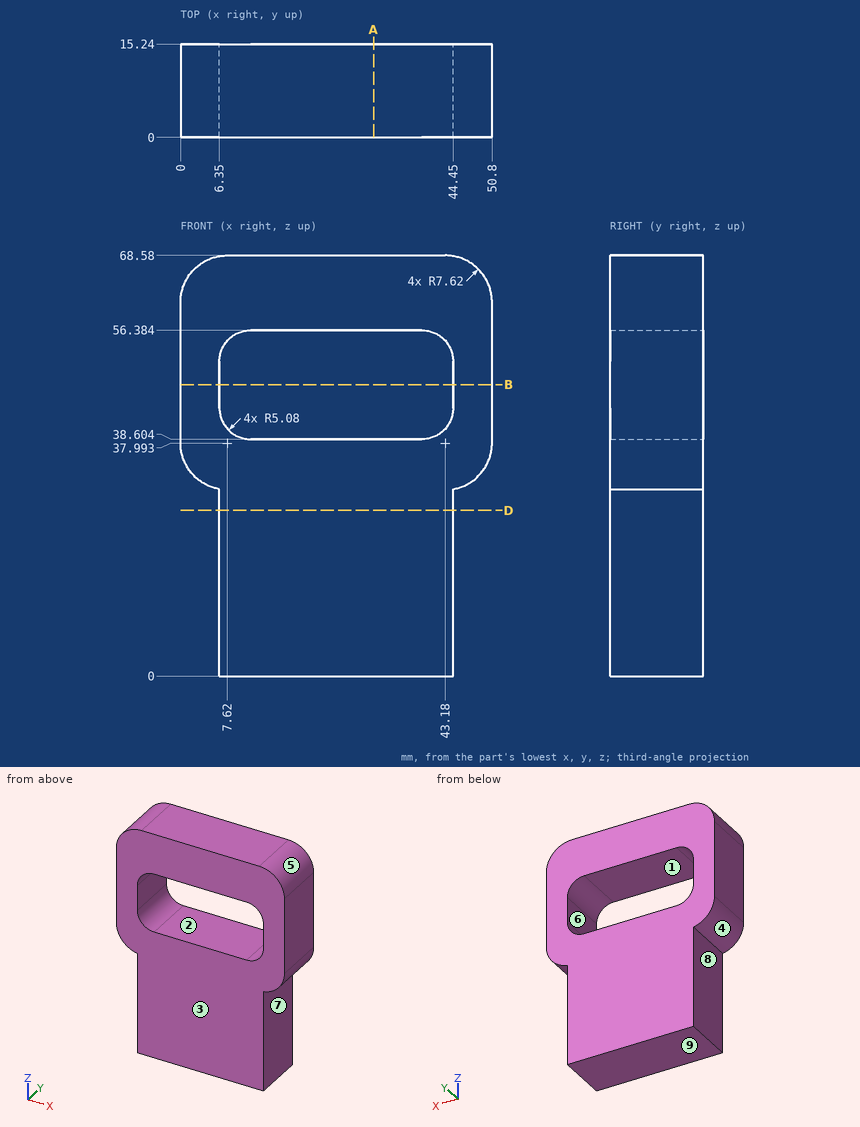
For this review, use the dimensioned drawing (mm, ordinates from the lowest corner) and the shaded views. A direction names the side the tool comes from. Give positions to 0.01 mm unless a question says otherwise; leave off trailing zeros. Loops run counter-clockwise (first coordinate to the right, second up) from the corner with the lowest first, then second, coordinate; pieces in that order, holes last. Notation, with made-up numbers: (64.25, -29) -> (82.25, -29) arc R12 cw to (82.25, -20) -> close; hole circle Ø4 at (78, 13). An arc over 180 degrees is marked (long way). Use CSV: the item, a comma, the result in double quotes.
1. Consider section D-D, the plane z = 27. Write out the cut boundary in (x, y).
Result:
outline,"(6.35, 0) -> (44.45, 0) -> (44.45, 15.24) -> (6.35, 15.24) -> close"
2. For P1, Ø5, axis at y = 5.5, z = 35, coming from the -X side; P2, Ø5, axis at x = 7.5, y = 5, coming from the -Z side; P3, Ø7.5, axis at y = 4, z = 18, coming from the +X side; P4, Ø1.5, axis at y = 11, z = 26, coming from the -X side, all flat-tipped, find the tip position at first contact; note any pin that passes through.
Result:
P1,"stops at x = 0.02"
P2,"stops at z = 0"
P3,"stops at x = 44.45"
P4,"stops at x = 6.35"
3. To check wall thickness, follow probe 1 along X at (y, z) = (14, 45); probe 2 along Z at (x, y) = (32.5, 2.25) (1 decimal); probe 3 along Z at (x, y) = (40, 8.5) (1 decimal). State the ranges of each line that lie inside material, in increasing order. Write a range as from..to.
Result:
probe 1,"x = 0..6.35, 44.45..50.8"
probe 2,"z = 0..38.6, 56.4..68.6"
probe 3,"z = 0..38.6, 56.3..68.6"
4. The part is to be moulded in two halves that separate along X. For the marked faces 1, 2, 3 and 4, say which applies: +X half, -X half, draft (parallel to the pull), parting line (faces both ways), or undercut.
Result:
face 1,"undercut"
face 2,"undercut"
face 3,"draft"
face 4,"-X half"
5. Consider section A-A, the plane x = 31.5. Write out the cut boundary in (y, z) (1 decimal).
Result:
outline,"(0, 0) -> (15.2, 0) -> (15.2, 38.6) -> (0, 38.6) -> close; (0, 56.4) -> (15.2, 56.4) -> (15.2, 68.6) -> (0, 68.6) -> close"
6. Consider section B-B, the plane z = 47.5. Write out the cut boundary in (x, y).
Result:
outline,"(0, 0) -> (6.35, 0) -> (6.35, 15.24) -> (0, 15.24) -> close; (44.45, 0) -> (50.8, 0) -> (50.8, 15.24) -> (44.45, 15.24) -> close"
7. Machinability: for the marked faces 5, 6, 7, 8 and 9, which of the approach directions +Z, -Z, +X, -X, +Y, -Y give a long, thin tool a straight path to every point of the face, cutting with its end or side? Answer none if there is none.
Result:
face 5,"+Z, +X, +Y, -Y"
face 6,"+Y, -Y"
face 7,"-Z, +X, +Y, -Y"
face 8,"-Z, -X, +Y, -Y"
face 9,"-Z, +X, -X, +Y, -Y"
